Here's how the part is built. I have some questions about the finished solid (model axes, mm). A direction names the side the tool comes from. Give positions to 0.01 mm unless a question says otherwise; leave off trailing zeros. Write each loop counter-clockwise with the first axis right and the second up, starting at its lowest first coordinate (ties: lowest second). Pieces come first, ordered by that corner, then holes. Notation, with made-up numbers: M 18,83 L 24,83 A20 cw 24,116 Z; hole C 61,-24 d5. An arc over 180 degrees is marked long. Answer as CSV lines item,"result". Start each with the question number.
Q1. Suppose I cut it at B-B (x = -2.5). Write out the boundary of the cut face in (y, z).
Q2. For pin 1 (1.4 mm diameter, centred on x = 55, z = -2, fed in from +Y); pin 2 (1.1 mm diameter, centred on x = 72, z = 1.5, fed in from +Y); pin 3 (0.7 mm diameter, centred on x = 71.5, z = 1.5, fed in from -Y), each with a flat end and sliding along its axis, tell me the tip position at first contact or that it passes through.
Q3. Suppose I cut it at C-C (x = 54.44). Write out the boundary of the cut face in (y, z).
Q4. Suppose I cut it at D-D (y = -7.75). Write out the boundary of the cut face in (x, z).
Q5. Suppose I cut it at A-A (z = -2.25). Write out the boundary of the cut face in (x, y), then the cut area to 3 significant figures.
Q6. If I drill on line 1 along Y through (x, z) = (63.1, 2.8); line 2 along Z through (x, y) = (54, -14.5); line 3 along Z through (x, y) = (24, -4.75), over which ranges is the centre line in solid material (lowest first)?
Q7. Thinking about a two-plate mould opening in Y: for faces 1 (the cylindrical face through (-15, -15, 2)), 2 (the flat face through (65, -30, 2)), 3 (the cylindrical face through (72.2, -15, 3.6)), which applies, +Y half, -Y half, draft (parallel to the pull), parting line (faces both ways), or undercut?
Q8. On a 3-axis mill with a long thin cutter (end or side, diameter ignored), from which of +Z, -Z, +X, -X, +Y, -Y can I reach the whole of each face in a straight line? I mean faces 4 (the flat face through (83, -15, 3.4)), 5 (the flat face through (5.4, -17, 1)), 6 (the flat face through (82, -21, -2)). Say none if no direction works.
```python
from build123d import *
from build123d.topology import SkipClean

# Parameters (mm, degrees)
BOSS_EXTRUDE1_DEPTH        = 5
CROQUIS3_W                 = 23
CROQUIS3_H                 = 12
CORTAR_EXTRUIR2_DEPTH      = 2.2
CORTAR_EXTRUIR3_DEPTH      = 91.182259896
CORTAR_EXTRUIR3_DEPTH_BACK = 91.182259896
CUT_EXTRUDE4_DEPTH         = 91.277350426
CUT_EXTRUDE4_DEPTH_BACK    = 2
CUT_EXTRUDE6_DEPTH         = 91.188691087
BOSS_EXTRUDE2_START        = 4.6
SKETCH9_W                  = 5
SKETCH9_H                  = 12
BOSS_EXTRUDE2_DEPTH        = 4.6
SKETCH10_R                 = 0.9
CUT_EXTRUDE7_DEPTH         = 8
CUT_EXTRUDE8_DEPTH         = 91.458609319


with BuildPart() as part:
    # Sketch1 → Boss-Extrude1 (new body)
    with BuildSketch(Plane(origin=(0, 0, 0), x_dir=(-1, 0, 0), z_dir=(0, 0, -1))):
        with BuildLine():
            Line((-70, 0), (-61, 0))
            ThreePointArc((-61, 0), (-35, -3.837363086), (-9, 0))
            Line((-9, 0), (0, 0))
            ThreePointArc((0, 0), (15, -15), (0, -30))
            Line((0, -30), (-9, -30))
            ThreePointArc((-9, -30), (-35, -26.162636914), (-61, -30))
            Line((-61, -30), (-70, -30))
            ThreePointArc((-70, -30), (-85, -15), (-70, 0))
        make_face()
        with BuildLine():
            Line((0, -11.4), (-5.4, -11.905))
            Line((-5.4, -11.905), (-5.4, -18.095))
            Line((-5.4, -18.095), (0, -18.6))
            ThreePointArc((0, -18.6), (3.6, -15), (0, -11.4))
        make_face(mode=Mode.SUBTRACT)
    extrude(amount=-BOSS_EXTRUDE1_DEPTH)

    # Croquis3 → Cortar-Extruir2 (cut)
    with BuildSketch(Plane(origin=(0, 0, 0), x_dir=(-1, 0, 0), z_dir=(0, 0, -1))):
        with Locations((-68.5, -15)):
            Rectangle(CROQUIS3_W, CROQUIS3_H)
    extrude(amount=-CORTAR_EXTRUIR2_DEPTH, mode=Mode.SUBTRACT)

    # Croquis4 → Cortar-Extruir3 (cut, two sides: drawn at the far end of the back side and taken through both)
    with BuildSketch(Plane(origin=(0, 0, 2.2), x_dir=(-1, 0, 0), z_dir=(0, 0, -1)).offset(-CORTAR_EXTRUIR3_DEPTH_BACK)):
        with BuildLine():
            Line((-66.2, -9.746429785), (-70.724590164, -12.416276944))
            ThreePointArc((-70.724590164, -12.416276944), (-72.2, -15), (-70.724590164, -17.583723056))
            Line((-70.724590164, -17.583723056), (-66.2, -20.253570215))
            ThreePointArc((-66.2, -20.253570215), (-57, -15), (-66.2, -9.746429785))
        make_face()
    extrude(amount=CORTAR_EXTRUIR3_DEPTH + CORTAR_EXTRUIR3_DEPTH_BACK, mode=Mode.SUBTRACT)

    # Sketch6 → Cut-Extrude4 (cut, two sides: drawn at the far end of the back side and taken through both)
    with BuildSketch(Plane.XY.offset(5).offset(-CUT_EXTRUDE4_DEPTH_BACK)):
        with BuildLine():
            Line((14.08705036, -12.406737159), (-1.12381295, -11.309587495))
            ThreePointArc((-1.12381295, -11.309587495), (-5.09, -15), (-1.12381295, -18.690412505))
            Line((-1.12381295, -18.690412505), (14.08705036, -17.593262841))
            ThreePointArc((14.08705036, -17.593262841), (16.5, -15), (14.08705036, -12.406737159))
        make_face()
    extrude(amount=CUT_EXTRUDE4_DEPTH + CUT_EXTRUDE4_DEPTH_BACK, mode=Mode.SUBTRACT)

    # Sketch8 → Cut-Extrude6 (cut, through all)
    with SkipClean():  # the faces are left unmerged after this step: merging them gives an invalid solid
        with BuildSketch(Plane.XY.offset(3)):
            with BuildLine():
                Line((-1.12381295, -11.309587495), (0, -11.4))
                ThreePointArc((0, -11.4), (-3.6, -15), (0, -18.6))
                Line((0, -18.6), (-1.12381295, -18.690412505))
                ThreePointArc((-1.12381295, -18.690412505), (-5.09, -15), (-1.12381295, -11.309587495))
            make_face()
        extrude(amount=-CUT_EXTRUDE6_DEPTH, mode=Mode.SUBTRACT)

    # Sketch9 → Boss-Extrude2 (add)
    with SkipClean():  # the faces are left unmerged after this step: merging them gives an invalid solid
        with BuildSketch(Plane(origin=(0, 0, 0), x_dir=(-1, 0, 0), z_dir=(0, 0, -1)).offset(BOSS_EXTRUDE2_START)):
            with BuildLine():
                Line((-83.747727085, -21), (-80, -21))
                Line((-80, -21), (-80, -9))
                Line((-80, -9), (-83.747727085, -9))
                ThreePointArc((-83.747727085, -9), (-85, -15), (-83.747727085, -21))
            make_face()
            with Locations((-54.5, -15)):
                Rectangle(SKETCH9_W, SKETCH9_H)
        extrude(amount=-BOSS_EXTRUDE2_DEPTH)

    # Sketch10 → Cut-Extrude7 (cut)
    with SkipClean():  # the faces are left unmerged after this step: merging them gives an invalid solid
        with BuildSketch(Plane(origin=(0, 0, -4.6), x_dir=(-1, 0, 0), z_dir=(0, 0, -1))):
            with Locations((-54.44, -15)):
                Circle(SKETCH10_R)
            with Locations(Location((-82.56, -15, 0), (0, 0, 180))):
                Circle(SKETCH10_R)
        extrude(amount=-CUT_EXTRUDE7_DEPTH, mode=Mode.SUBTRACT)

    # Sketch11 → Cut-Extrude8 (cut, through all)
    with SkipClean():  # the faces are left unmerged after this step: merging them gives an invalid solid
        with BuildSketch(Plane.XY.offset(3)):
            with BuildLine():
                Line((4.96, -14.25), (12.46, -14.25))
                ThreePointArc((12.46, -14.25), (13.21, -15), (12.46, -15.75))
                Line((12.46, -15.75), (4.96, -15.75))
                Line((4.96, -15.75), (4.96, -14.25))
            make_face()
        extrude(amount=-CUT_EXTRUDE8_DEPTH, mode=Mode.SUBTRACT)


solid = part.part
```
Resolved:
1,outline,"M -29.79,0 L -18.53,0 L -18.53,5 L -29.79,5 Z; M -11.47,0 L -0.21,0 L -0.21,5 L -11.47,5 Z"
2,pin 1,"y = -9"
2,pin 2,"y = -0.07"
2,pin 3,"y = -29.96"
3,outline,"M -28.29,0 L -21,0 L -21,-4.6 L -15.9,-4.6 L -15.9,3.4 L -14.1,3.4 L -14.1,-4.6 L -9,-4.6 L -9,0 L -1.71,0 L -1.71,5 L -28.29,5 Z"
4,outline,"M -13.13,0 L 83.13,0 L 83.13,5 L -13.13,5 Z"
5,outline,"M 52,-21 L 57,-21 L 57,-9 L 52,-9 Z; M 80,-21 L 83.75,-21 A15 ccw 83.75,-9 L 80,-9 Z; hole C 54.44,-15 d1.8; hole C 82.56,-15 d1.8"
5,area,"110 mm^2"
6,line 1,"-30 to -21.1, -8.9 to 0"
6,line 2,"3.4 to 5"
6,line 3,"0 to 5"
7,face 1,"parting line"
7,face 2,"-Y half"
7,face 3,"undercut"
8,face 4,"-Z"
8,face 5,"+Z, -Z"
8,face 6,"-Z, +X, -X, -Y"
